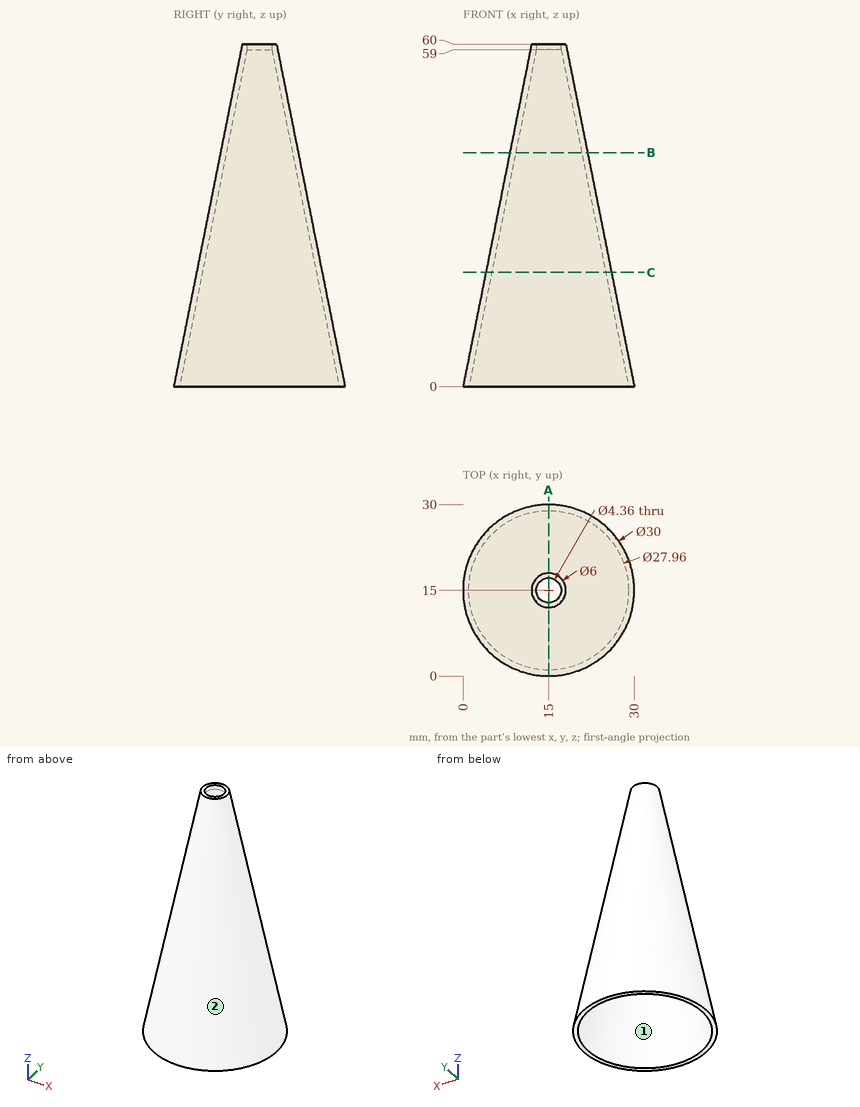
The figure shows three views and two pictorial views of one solid part (mm, origin at its lowest corner). Answer the questions. Give positions to 0.01 mm unless a question says otherwise; leave off trailing zeros. Loops run counter-clockwise (first coordinate to the right, second up) from the corner with the lowest first, then second, coordinate; pieces in that order, holes last. Notation, with made-up numbers: (59.5, 70.25) - (96.5, 70.25) arc R33 cw to (96.5, 107.25) - close; hole circle Ø10 at (25.25, 5.5). An arc over 180 degrees is marked (long way). Answer in a Markdown table with one row per item.
(1) Consider L1, parallel to X at y = 13.5, z = 37; L2, parallel to X at y = 23.5, z = 7 (1 decimal); L3, parallel to Y at x = 13, z = 5 (1 decimal). Determine where each line is inside the solid, lowest interval first. Write a range as [from, to].
Results list:
| item | result |
|---|---|
| L1 | x = [7.55, 8.59], [21.41, 22.45] |
| L2 | x = [4.4, 5.7], [24.3, 25.6] |
| L3 | y = [1.1, 2.2], [27.8, 28.9] |
(2) Section B-B (z = 41) is taken. Give the vertices of the cut face in (x, y).
Results list:
| item | result |
|---|---|
| outline | circle Ø13.6 at (15, 15); hole circle Ø11.56 at (15, 15) |
(3) Section C-C (z = 20) is taken. Give the vertices of the cut face in (x, y).
Results list:
| item | result |
|---|---|
| outline | circle Ø22 at (15, 15); hole circle Ø19.96 at (15, 15) |
(4) Section A-A (x = 15) is taken. Give the vertices of the cut face in (y, z), and give its area (3 significant figures).
Results list:
| item | result |
|---|---|
| outline | (0, 0) - (1.02, 0) - (12.82, 59) - (12.82, 60) - (12, 60) - close; (17.18, 59) - (28.98, 0) - (30, 0) - (18, 60) - (17.18, 60) - close |
| area | 122 mm² |
(5) Flat-ended cylindrical pins translate along their axes: pin 1 Ø5 at (x, y) = (26, 9) entering from -Z; pin 2 Ø5 at (x, z) = (23, 28.5) entering from +Y; pin 3 Ø4 at (y, z) = (10, 36.5) entering from -X (1 decimal); pin 4 Ø8 at (x, z) = (21, 33.5) entering from +Y (1 decimal). Find the tip coordinate at first contact, or state that the pin passes through.
Results list:
| item | result |
|---|---|
| pin 1 | stops at z = 0 |
| pin 2 | stops at y = 22.6 |
| pin 3 | stops at x = 7.8 |
| pin 4 | stops at y = 23.3 |
(6) For a pull along X with two mould halves and no side action, classify the marked faces 1 and 2 as pulls with the +X half, pulls with the -X half, needs draft (parallel to the pull), parting line crosses it, or undercut.
Results list:
| item | result |
|---|---|
| face 1 | undercut |
| face 2 | parting line crosses it |
